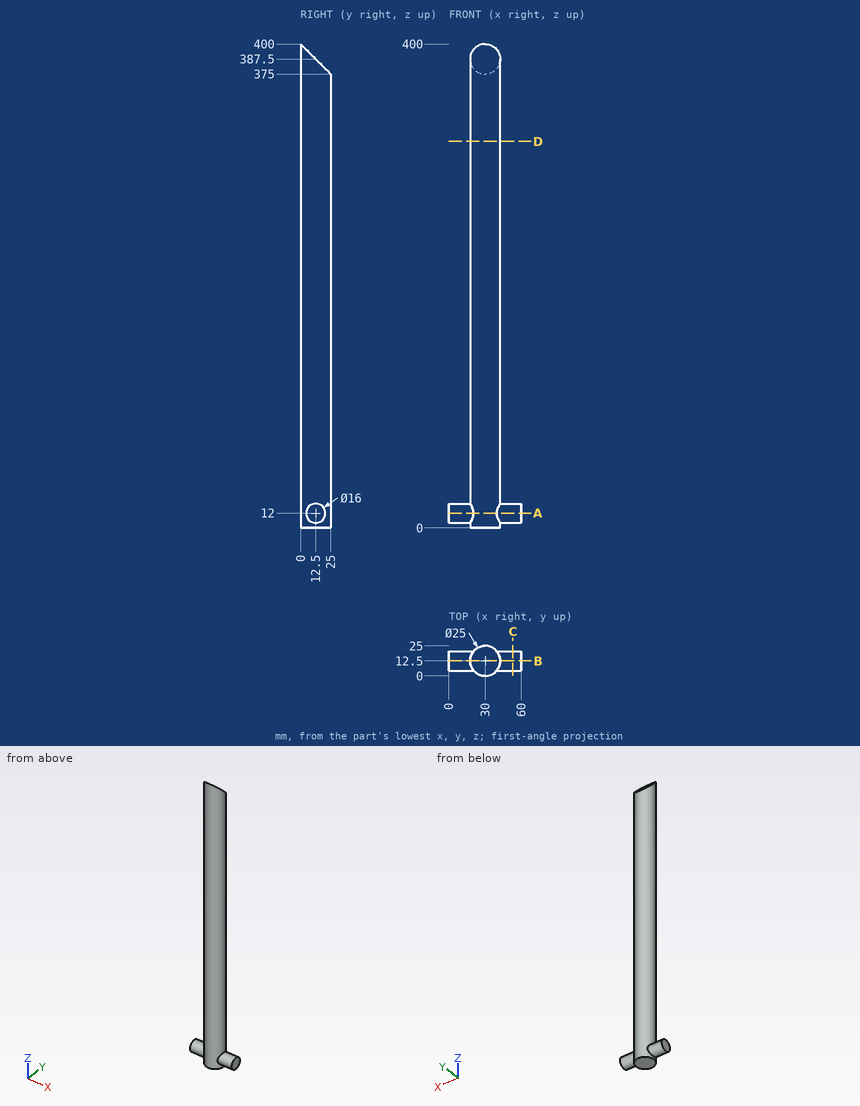
Source: three-view drawing plus pictorial views. Frame: mm from the lowest corner of the part. Round coordinates to 2 decimals unless told otherwise and drop trailing zeros. Write each loop counter-clockwise with the first axis right and the second up, starting at its lowest first coordinate (ties: lowest second). Pieces come first, ordered by that corner, then holes. Notation, with made-up numbers: M 55.5,-33.75 L 77.5,-33.75 A20 cw 77.5,-11.75 Z; hole C 53,18 d10. An arc over 180 degrees is marked long. Use CSV: the item, a comma, the result in double quotes. Start each with the question number.
Q1. Cut plane C-C on x = 53. Output: boundary loops of the cut face in (y, z), plus the area to 3 significant figures.
Q2. First-contact query: P1, Ø10, axis at y = 14, z = 159.5, coming from the +X side; P2, Ø1, axis at x = 33, z = 349.5, coming from the +Y side; P3, Ø12, axis at x = 39.5, z = 218.5, coming from the +Y side. Flat tips, straight axial feed; report the tip coordinate or a pass-through.
Q3. Cut plane A-A on z = 12. Output: boundary loops of the cut face in (x, y).
Q4. Cut plane B-B on y = 12.5. Output: boundary loops of the cut face in (x, z).
Q5. Cut plane D-D on z = 319.5. Output: boundary loops of the cut face in (x, y), plus the area to 3 significant figures.
Q6. Line query: line 1 (X direction, y = 15.25, z = 321); line 2 (X direction, y = 13.5, z = 316); line 3 (Y direction, x = 37.5, z = 321). Output: solid intervals per line, ascending. Write a range as from..to.
Results found:
1,outline,"C 12.5,12 d16"
1,area,"201 mm^2"
2,P1,"x = 42.5"
2,P2,"y = 24.75"
2,P3,"y = 24.5"
3,outline,"M 0,4.5 L 20.4,4.5 A12.5 ccw 39.6,4.5 L 60,4.5 L 60,20.5 L 39.6,20.5 A12.5 ccw 20.4,20.5 L 0,20.5 Z"
4,outline,"M 0,4 L 17.5,4 L 17.5,0 L 42.5,0 L 42.5,4 L 60,4 L 60,20 L 42.5,20 L 42.5,387.5 L 17.5,387.5 L 17.5,20 L 0,20 Z"
5,outline,"C 30,12.5 d25"
5,area,"491 mm^2"
6,line 1,"17.81..42.19"
6,line 2,"17.54..42.46"
6,line 3,"2.5..22.5"
